Could you check a few things on this model? Use its own coordinates, in mm. A direction names the side the tool comes from. Round coordinates to 2 decimals unless told otherwise and drop trailing zeros. Order: outer loops, then holes, each group sorted by start corner. A loop starts at its lowest first (then second) coordinate and runs counter-clockwise, first axis right, second up. Notation, with made-up numbers: (8, 22) - (62, 22) arc R12 cw to (62, 37) - close; hole circle Ø5 at (15, 1). An arc over 180 degrees is marked (long way). Use one line per item in the form item = value.
from build123d import *

# Parameters (mm, degrees)
SKETCH1_W           = 280
SKETCH1_H           = 60
BOSS_EXTRUDE1_DEPTH = 3
SKETCH1_9_W         = 280
SKETCH1_9_H         = 0.5
CUT_EXTRUDE1_DEPTH  = 1
BOSS_EXTRUDE2_DEPTH = 280
SKETCH3_W           = 0.15
SKETCH3_H           = 0.5
CUT_EXTRUDE5_DEPTH  = 280


with BuildPart() as part:
    # Sketch1 → Boss-Extrude1 (new body)
    with BuildSketch(Plane(origin=(0, 0, 0), x_dir=(1, 0, 0), z_dir=(0, 1, 0))):
        Rectangle(SKETCH1_W, SKETCH1_H)
    extrude(amount=-BOSS_EXTRUDE1_DEPTH)

    # Sketch1_9 → Cut-Extrude1 (cut)
    with BuildSketch(Plane(origin=(0, 0, 0), x_dir=(1, 0, 0), z_dir=(0, 1, 0))):
        with Locations((0, 27.25)):
            Rectangle(SKETCH1_9_W, SKETCH1_9_H)
    cut_extrude1 = extrude(amount=-CUT_EXTRUDE1_DEPTH, mode=Mode.SUBTRACT)

    # Mirror1: Cut-Extrude1 across plane
    add(cut_extrude1.mirror(Plane.XY), mode=Mode.SUBTRACT)

    # Sketch2 → Boss-Extrude2 (add)
    with BuildSketch(Plane(origin=(140, 0, 0), x_dir=(0, 0, -1), z_dir=(1, 0, 0))):
        Polygon((0, 0.5), (2, 0.5), (2, 0), (-2, 0), (-2, 0.5), align=None)
    extrude(amount=-BOSS_EXTRUDE2_DEPTH)

    # Sketch3 → Cut-Extrude5 (cut)
    with BuildSketch(Plane(origin=(140, 0, 0), x_dir=(0, 0, -1), z_dir=(1, 0, 0))):
        with Locations((0.075, 0.25)):
            Rectangle(SKETCH3_W, SKETCH3_H)
        with Locations((-0.075, 0.25)):
            Rectangle(SKETCH3_W, SKETCH3_H)
    extrude(amount=-CUT_EXTRUDE5_DEPTH, mode=Mode.SUBTRACT)


solid = part.part
Item 1: Will this pin go through, and if not, where does the flat tip stop? P1, Ø3, axis at x = 57.5, z = -29, coming from the +Y side.
Found:
P1 = 0
Item 2: I need wall thicknesses on L1, parallel to Z at x = -71.5, y = -0.4; L2, parallel to Y at x = -35, z = 18.5. Which ranges of each line are inside material? Lowest first, please.
Found:
L1 = -30 to -27.5, -27 to 27, 27.5 to 30
L2 = -3 to 0
Item 3: Imagine slicing it at B-B on z = 18. Please give me the cut outline in (x, y), plus the area to 3 significant figures.
Found:
outline = (-140, -3) - (140, -3) - (140, 0) - (-140, 0) - close
area = 840 mm2
Item 4: For faces 1 (the face through (-2, 0, -15)), 2 (the face through (-2, 0, 14)), 3 (the face through (-2, -3, 0)), which set-ups out of +Z, -Z, +X, -X, +Y, -Y let a thin tool reach every point of the face, with its end or its side?
Found:
face_1 = -Z, +X, -X, +Y
face_2 = +Z, +X, -X, +Y
face_3 = +Z, -Z, +X, -X, -Y
Item 5: Imagine slicing it at A-A on x = -47. Please give me the cut outline in (y, z).
Found:
outline = (-3, -30) - (0, -30) - (0, -27.5) - (-1, -27.5) - (-1, -27) - (0, -27) - (0, -2) - (0.5, -2) - (0.5, -0.15) - (0, -0.15) - (0, 0.15) - (0.5, 0.15) - (0.5, 2) - (0, 2) - (0, 27) - (-1, 27) - (-1, 27.5) - (0, 27.5) - (0, 30) - (-3, 30) - close
